Here's how the part is built. I have some questions about the finished solid (model axes, mm). A direction names the side the tool comes from. Round coordinates to 2 decimals unless told otherwise and drop trailing zeros. Loops run counter-clockwise (first coordinate to the right, second up) from the corner with the lowest first, then second, coordinate; pieces in that order, holes last. Notation, with made-up numbers: (10, 61.25) - (32, 61.25) arc R28 cw to (32, 86.25) - close; hole circle Ø4 at (8, -24.5). An arc over 180 degrees is marked (long way). Answer as a JSON object with one key per item and string values. Group by question number.
1) I want a section at C-C, the plane x = 32. Please give me the cut outline in (y, z), then the cut area to 3 significant figures.
2) Will these pins go through, and if not, where does the flat tip stop? P1, Ø6, axis at y = 56.5, z = -3.5, coming from the -X side; P2, Ø3, axis at y = -41.5, z = 0, coming from the +X side; P3, Ø1, axis at x = 20, z = -3.5, coming from the +Y side; P4, Ø19.5, axis at x = 0, y = 0, coming from the +Z side.
3) If I drill on line 1 along Y through (x, z) = (35, -1.5); line 2 along Y through (x, z) = (-0.5, 4); line 3 along X through (y, z) = (-54.5, 4), over which ranges is the centre line in solid material (lowest first)? Write a range as [from, to].
4) I want a section at A-A, the plane x = 0. Please give me the cut outline in (y, z).
5) I want a section at D-D, the plane y = -33. Please give me the cut outline in (x, z), then the cut area to 3 significant figures.
6) Which directions (+Z, -Z, +X, -X, +Y, -Y) give clear straight access to the entire face, cutting with the end or side of a thin tool? Please do faces 4 (the face through (33, -8, 0)), 5 (the face through (-8, 63, 0)), 6 (the face through (-8, -64, 0)), 7 (the face through (33, 8, 0)).
7) If we mould it in two halves opening along Y, with no side actions, what happens to faces 1 (the face through (8, 63, 0)), 2 (the face through (-8.49, 0.37, -0.11)), 3 (the face through (17.761, 17.594, 0.112))? For each: pulls with the +Y half, pulls with the -Y half, needs draft (parallel to the pull), parting line crosses it, or undercut.
8) I want a section at B-B, the plane z = 5. Please give me the cut outline in (x, y), then the cut area to 3 significant figures.
from build123d import *

# Parameters (mm, degrees)
SKETCH1_R               = 25
SKETCH1_R_2             = 8.5
BOSS_EXTRUDE1_DEPTH     = 8
SKETCH2_W               = 16
SKETCH2_H               = 76.314561435
BOSS_EXTRUDE2_DEPTH     = 8
SKETCH3_W               = 16
SKETCH3_H               = 76.314561435
BOSS_EXTRUDE3_DEPTH     = 8
SKETCH4_W               = 16.314561435
SKETCH4_H               = 16
BOSS_EXTRUDE4_DEPTH     = 8
CUT_EXTRUDE1_DEPTH      = 109
CUT_EXTRUDE1_DEPTH_BACK = 109
SKETCH5_W               = 48
SKETCH5_H               = 0.5
FILLET1_R               = 5


with BuildPart() as part:
    # Sketch1 → Boss-Extrude1 (new, symmetric)
    with BuildSketch(Plane.XY):
        Circle(SKETCH1_R)
        Circle(SKETCH1_R_2, mode=Mode.SUBTRACT)
    extrude(amount=BOSS_EXTRUDE1_DEPTH, both=True)

    # Sketch2 → Boss-Extrude2 (add, symmetric)
    with BuildSketch(Plane.XY):
        with Locations((0, 61.842719282)):
            Rectangle(SKETCH2_W, SKETCH2_H)
    extrude(amount=BOSS_EXTRUDE2_DEPTH, both=True)

    # Sketch3 → Boss-Extrude3 (add, symmetric)
    with BuildSketch(Plane.XY):
        with Locations((0, -61.842719282)):
            Rectangle(SKETCH3_W, SKETCH3_H)
    extrude(amount=BOSS_EXTRUDE3_DEPTH, both=True)

    # Sketch4 → Boss-Extrude4 (add, symmetric)
    with BuildSketch(Plane.XY):
        with Locations((31.842719282, 0)):
            Rectangle(SKETCH4_W, SKETCH4_H)
    extrude(amount=BOSS_EXTRUDE4_DEPTH, both=True)

    # Sketch5 → Cut-Extrude1 (cut, two sides: drawn at the far end of the back side and taken through both)
    with BuildSketch(Plane.XY.offset(-CUT_EXTRUDE1_DEPTH_BACK)):
        with Locations((26, 0)):
            Rectangle(SKETCH5_W, SKETCH5_H)
    extrude(amount=CUT_EXTRUDE1_DEPTH + CUT_EXTRUDE1_DEPTH_BACK, mode=Mode.SUBTRACT)

    # Fillet1
    fillet1_edges = [part.edges().sort_by_distance(p)[0] for p in [
        (8, 23.685438565, 0),
        (-8, 23.685438565, 0),
        (8, -23.685438565, 0),
        (-8, -23.685438565, 0),
        (23.685438565, -8, 0),
        (23.685438565, 8, 0),
    ]]
    fillet(fillet1_edges, radius=FILLET1_R)


solid = part.part
Outcome:
{
 "1": {"outline": "(-8, -8) - (-0.25, -8) - (-0.25, 8) - (-8, 8) - close; (0.25, -8) - (8, -8) - (8, 8) - (0.25, 8) - close", "area": "248 mm^2"},
 "2": {"P1": "x = -8", "P2": "x = 8", "P3": "y = 15.64", "P4": "z = 8"},
 "3": {"line 1": "[-8, -0.25], [0.25, 8]", "line 2": "[-100, -8.49], [8.49, 100]", "line 3": "[-8, 8]"},
 "4": {"outline": "(-100, -8) - (-8.5, -8) - (-8.5, 8) - (-100, 8) - close; (8.5, -8) - (100, -8) - (100, 8) - (8.5, 8) - close"},
 "5": {"outline": "(-8, -8) - (8, -8) - (8, 8) - (-8, 8) - close", "area": "256 mm^2"},
 "6": {"face 4": "+Z, -Z, +X, -Y", "face 5": "+Z, -Z, -X, +Y", "face 6": "+Z, -Z, -X, -Y", "face 7": "+Z, -Z, +X, +Y"},
 "7": {"face 1": "needs draft", "face 2": "undercut", "face 3": "pulls with the +Y half"},
 "8": {"outline": "(-10.83, -22.53) arc R5 cw to (-8, -27.04) - (-8, -100) - (8, -100) - (8, -27.04) arc R5 cw to (10.83, -22.53) arc R25 ccw to (22.53, -10.83) arc R5 cw to (27.04, -8) - (40, -8) - (40, -0.25) - (8.5, -0.25) arc R8.5 cw (long way) to (8.5, 0.25) - (40, 0.25) - (40, 8) - (27.04, 8) arc R5 cw to (22.53, 10.83) arc R25 ccw to (10.83, 22.53) arc R5 cw to (8, 27.04) - (8, 100) - (-8, 100) - (-8, 27.04) arc R5 cw to (-10.83, 22.53) arc R25 ccw to start", "area": "4,390 mm^2"}
}
